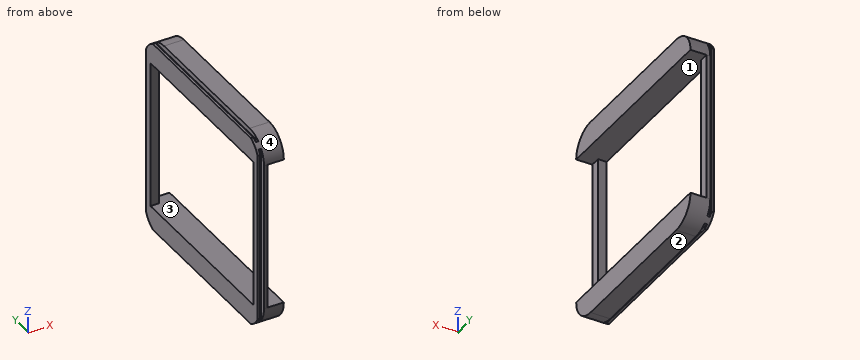
from build123d import *

# Parameters (mm, degrees)
F0_W      = 160
F0_H      = 160
F1_DEPTH  = 20
F2_R      = 20
F3_W      = 144
F3_H      = 120
F4_DEPTH  = 60
F5_W      = 160
F5_H      = 120
F6_DEPTH  = 13
F7_W      = 2
F7_H      = 2
F8_DEPTH  = 153.4
F9_W      = 2
F9_H      = 2
F9_W_2    = 3.241547
F9_H_2    = 2.78797
F10_DEPTH = 165


with BuildPart() as f1:
    # F0 (on Right) → F1 (new body)
    with BuildSketch(Plane.YZ):
        with Locations((27.151147, 20.321211)):
            Rectangle(F0_W, F0_H)
    extrude(amount=F1_DEPTH)

    # F2
    f2_edges = [f1.edges().sort_by_distance(p)[0] for p in [
        (10, -52.848853, 100.321211),
        (10, 107.151147, 100.321211),
        (10, -52.848853, -59.678789),
        (10, 107.151147, -59.678789),
    ]]
    fillet(f2_edges, radius=F2_R)

    # F3 (on face) → F4 (cut)
    with BuildSketch(Plane.YZ.offset(20)):
        with Locations((27.151147, 20.321211)):
            Rectangle(F3_W, F3_H)
    extrude(amount=-F4_DEPTH, mode=Mode.SUBTRACT)

    # F5 (on face) → F6 (cut)
    with BuildSketch(Plane.YZ.offset(20)):
        with Locations((27.151147, 20.321211)):
            Rectangle(F5_W, F5_H)
    extrude(amount=-F6_DEPTH, mode=Mode.SUBTRACT)

    # F7 (on face) → F8 (cut)
    with BuildSketch(Plane.XY.offset(100.321211)):
        Polygon((2, -52.848853), (2, -57.705119), (4, -57.705119), (4, -48.848853), (2, -48.848853), (2, -50.848853), align=None)
        with Locations((1, -51.848853)):
            Rectangle(F7_W, F7_H)
        Polygon((2, 103.151147), (4, 103.151147), (4, 113.693945), (2, 113.693945), (2, 107.151147), (2, 105.151147), align=None)
        with Locations((1, 106.151147)):
            Rectangle(F7_W, F7_H)
    extrude(amount=-F8_DEPTH, mode=Mode.SUBTRACT)

    # F9 (on face) → F10 (cut)
    with BuildSketch(Plane(origin=(0, 107.151147, 0), x_dir=(-1, 0, 0), z_dir=(0, 1, 0))):
        Polygon((-4, 96.321211), (-2, 96.321211), (-2, 98.321211), (-2, 100.321211), (-2, 102.704816), (-4, 102.704816), align=None)
        with Locations((-1, 99.321211)):
            Rectangle(F9_W, F9_H)
        Polygon((-2, -57.678789), (-2, -55.678789), (-4, -55.678789), (-4, -64.467512), (-2, -64.467512), (-2, -60.466759), align=None)
        with Locations((-0.379227, -59.072774)):
            Rectangle(F9_W_2, F9_H_2)
    extrude(amount=-F10_DEPTH, mode=Mode.SUBTRACT)


solid = f1.part
Design review of the part built by this model. Coordinates are the model's own, in mm. Face numbers are marked on the shaded views. Round coordinates to 2 decimals unless told otherwise and drop trailing zeros. Write each loop counter-clockwise with the first axis right and the second up, starting at its lowest first coordinate (ties: lowest second). Pieces come first, ordered by that corner, then holes.
Item 1: Consider section C-C on x = 12. Give the boundary of the cut face in (y, z).
Item 2: Wall thickness on L1, parallel to Y at x = 1.75, z = -38; L2, parallel to Z at x = 9, y = 10; L3, parallel to Y at x = 6.25, z = 30: over which ranges is each line inside the solid? List them lowest first.
Item 3: Draft analysis for pull direction Y (two halves, no side actions). For the marked faces 1, 2, 3 and 4, state which applies: released by +Y, released by -Y, zero draft, split by the parting line, or undercut.
Item 4: Consider section A-A on y = -9.5. Give the boundary of the cut face in (x, z).
Item 5: Consider section B-B on z = -21. Give the boundary of the cut face in (x, y).
Item 6: For pin 1 Ø0.6 at (x, y) = (3, -2) entering from +Z; pin 2 Ø1 at (x, y) = (1, 36.5) entering from +Z; pin 3 Ø2 at (y, z) = (-50, 37) entering from +X, all flat-tipped, find the tip position at first contact; note any pin that passes through.
Check values:
1. outline: (-52.85, -39.68) arc R20 ccw to (-32.85, -59.68) - (87.15, -59.68) arc R20 ccw to (107.15, -39.68) - close; (-52.85, 80.32) - (107.15, 80.32) arc R20 ccw to (87.15, 100.32) - (-32.85, 100.32) arc R20 ccw to start
2. L1: y = -50.85 to -44.85, 99.15 to 105.15
2. L2: z = -59.68 to -39.68, 80.32 to 100.32
2. L3: y = -52.85 to -44.85, 99.15 to 107.15
3. face 1: undercut
3. face 2: zero draft
3. face 3: undercut
3. face 4: released by -Y
4. outline: (0, -57.68) - (2, -57.68) - (2, -55.68) - (4, -55.68) - (4, -59.68) - (20, -59.68) - (20, -39.68) - (0, -39.68) - close; (0, 80.32) - (20, 80.32) - (20, 100.32) - (4, 100.32) - (4, 96.32) - (2, 96.32) - (2, 98.32) - (0, 98.32) - close
5. outline: (0, -50.85) - (2, -50.85) - (2, -48.85) - (4, -48.85) - (4, -52.85) - (7, -52.85) - (7, -44.85) - (0, -44.85) - close; (0, 99.15) - (7, 99.15) - (7, 107.15) - (4, 107.15) - (4, 103.15) - (2, 103.15) - (2, 105.15) - (0, 105.15) - close
6. pin 1: stops at z = 96.32
6. pin 2: stops at z = 98.32
6. pin 3: stops at x = 7
